Source: three-view drawing plus pictorial views. Frame: mm from the lowest corner of the part. Coordinates: 2 decimals unless noted, no trailing zeros. Write each loop counter-clockwise with the first axis right and the second up, starting at its lowest first coordinate (ties: lowest second). Pieces come first, ordered by that corner, then holes. Notation, with made-up numbers: (89, -4) - (118, -4) arc R12 cw to (118, 0) - close; hole circle Ø2 at (-27, 64). An arc over 180 degrees is marked (long way). Put each result on its own line as item: value. Start each with the question number.
1. Cut plane D-D, the plane z = 50.8. Return loops of the section in (x, y) (3 decimals).
2. Pull-direction query (X, two-part tool) for the marked faces 1, 2 and 3; classes: released by +X, released by -X, zero draft, split by the parting line, or undercut.
3. Cut plane A-A, the plane x = 285.75. Return loops of the section in (y, z) (3 decimals), and give its area (3 significant figures).
4. Pin query (flat end, axial travel): pin 1 (12 mm diameter, centred on x = 375, z = 396, fed in from -Y); pin 2 (1.5 mm diameter, centred on x = 475, z = 158, fed in from -Y); pin 3 (10 mm diameter, centred on x = 96, z = 655, fed in from -Y). Return the tip coordinate at first contact, or that it passes through.
5. Line query: line 1 (X direction, y = 294.5, z = 380.5); line 2 (Z direction, x = 285.75, y = 4.5) (3 decimals); line 3 (Z direction, x = 183.5, y = 517.5). Output: solid intervals per line, ascending.
6. Cut plane C-C, the plane x = 418. Return loops of the section in (y, z).
7. Cut plane B-B, the plane y = 434.5. Return loops of the section in (x, z), and give its area (3 significant figures).
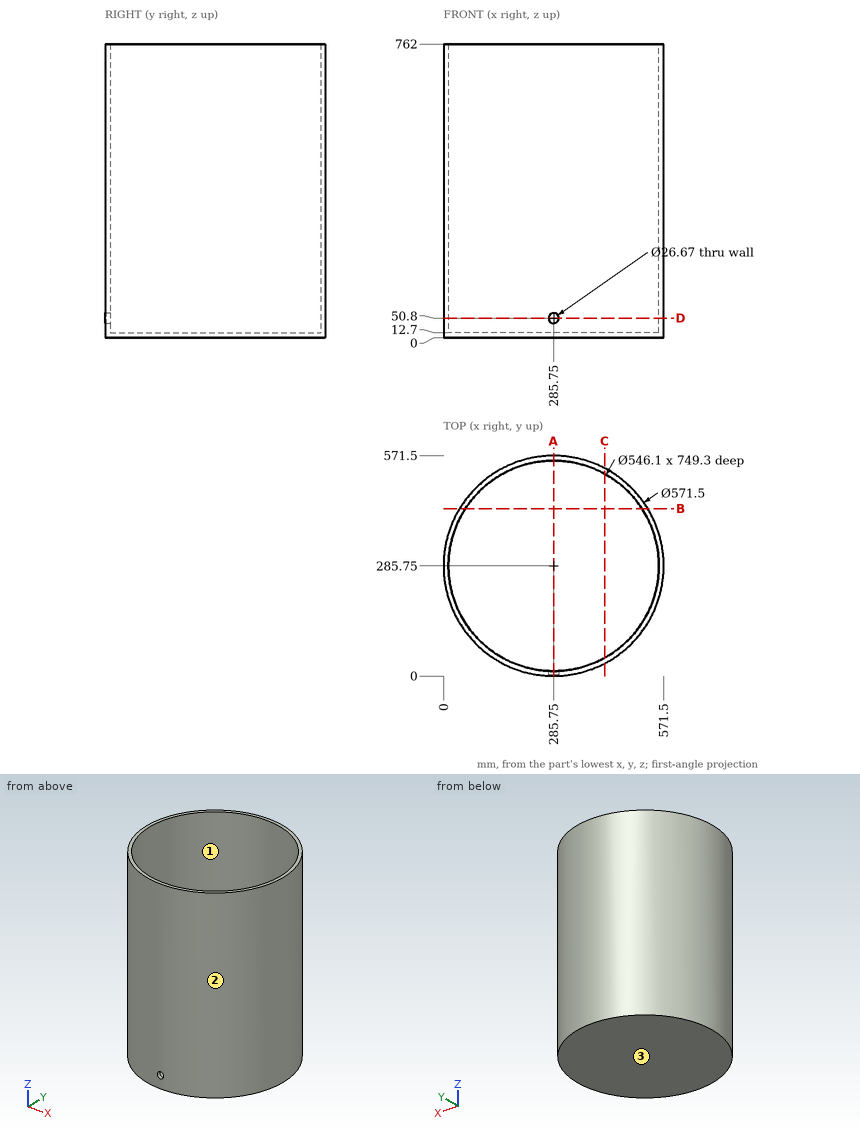
Report:
1. outline: (272.415, 0.311) - (272.415, 13.026) arc R273.05 cw (long way) to (299.085, 13.026) - (299.085, 0.311) arc R285.75 ccw (long way) to start
2. face 1: undercut
2. face 2: split by the parting line
2. face 3: zero draft
3. outline: (0, 0) - (571.5, 0) - (571.5, 762) - (558.8, 762) - (558.8, 12.7) - (12.7, 12.7) - (12.7, 37.465) - (0, 37.465) - close; (0, 64.135) - (12.7, 64.135) - (12.7, 762) - (0, 762) - close
3. area: 26,000 mm^2
4. pin 1: stops at y = 12.4
4. pin 2: stops at y = 70.99
4. pin 3: stops at y = 67.76
5. line 1: x = 0.13 to 12.84, 558.66 to 571.37
5. line 2: z = 0 to 37.465, 64.135 to 762
5. line 3: z = 0 to 12.7
6. outline: (32.45, 0) - (539.05, 0) - (539.05, 762) - (524.64, 762) - (524.64, 12.7) - (46.86, 12.7) - (46.86, 762) - (32.45, 762) - close
7. outline: (41.77, 0) - (529.73, 0) - (529.73, 762) - (514.73, 762) - (514.73, 12.7) - (56.77, 12.7) - (56.77, 762) - (41.77, 762) - close
7. area: 28,700 mm^2
